Job drawing, mm, ordinate dimensions from the low corner. One solid piece. A direction names the side the tool comes from. Round coordinates to 2 decimals unless told otherwise and drop trailing zeros. Order: outer loops, then holes, each group sorted by start corner. A loop starts at its lowest first (then second) coordinate and runs counter-clockwise, first axis right, second up. Notation, with made-up numbers: (8.5, 50) -> (49.5, 50) arc R16 cw to (49.5, 77) -> close; hole circle Ø5 at (70, 8.25). An arc over 180 degrees is marked (long way). Answer as a JSON object with one key per item and string values. Group by question number.
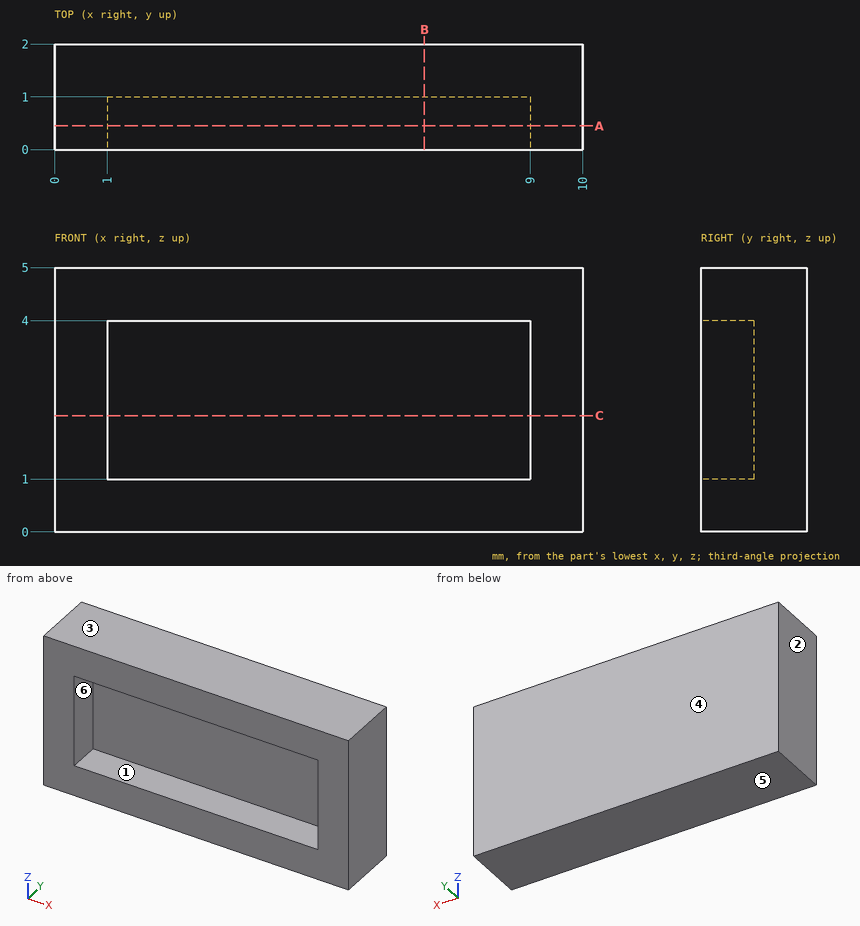
Q1. Band-saw the part on C-C (z = 2.2). List the corners of the cut face in (x, y).
Q2. Band-saw the part on B-B (x = 7). List the corners of the cut face in (y, z), plus the area to 3 significant figures.
Q3. Two-plate mould, pull along Z, no slides. Class the marked faces 3, 4, 5 and 6: +Z half, -Z half, draft (parallel to the pull), parting line (faces both ways), or undercut.
Q4. Band-saw the part on A-A (y = 0.45). List the corners of the cut face in (x, z), plus the area to 3 significant figures.
Q5. Wall check: line 1 (X direction, y = 0.65, z = 1.35); line 2 (Z direction, x = 2.25, y = 0.2); line 3 (Y direction, x = 4.5, z = 3.4). Give the ranges that are in metal, low to high. Write a range as [from, to].
Q6. Which spindle directions (+Z, -Z, +X, -X, +Y, -Y) get a long thin tool onto all of the face, cutting with end or side? Do the marked faces 1 and 2. Say none if no direction does.
Q7. Drop a flat-ended pin along its axis: pin 1 Ø0.9 at (x, z) = (5, 2) entering from -Y. Give the stop position or say it passes through.
Completed:
{
 "1": {"outline": "(0, 0) -> (1, 0) -> (1, 1) -> (9, 1) -> (9, 0) -> (10, 0) -> (10, 2) -> (0, 2) -> close"},
 "2": {"outline": "(0, 0) -> (2, 0) -> (2, 5) -> (0, 5) -> (0, 4) -> (1, 4) -> (1, 1) -> (0, 1) -> close", "area": "7.00 mm2"},
 "3": {"face 3": "+Z half", "face 4": "draft", "face 5": "-Z half", "face 6": "undercut"},
 "4": {"outline": "(0, 0) -> (10, 0) -> (10, 5) -> (0, 5) -> close; hole (1, 1) -> (9, 1) -> (9, 4) -> (1, 4) -> close", "area": "26.0 mm2"},
 "5": {"line 1": "[0, 1], [9, 10]", "line 2": "[0, 1], [4, 5]", "line 3": "[1, 2]"},
 "6": {"face 1": "-Y", "face 2": "+Z, -Z, -X, +Y, -Y"},
 "7": {"pin 1": "y = 1"}
}
